```python
from build123d import *

# Parameters (mm, degrees)
SKETCH1_R               = 31.877
SKETCH1_R_2             = 2.159
BOSS_EXTRUDE1_DEPTH     = 5.08
BOSS_EXTRUDE4_START     = -5.08
BOSS_EXTRUDE4_DEPTH     = 5.08
CUT_EXTRUDE1_DEPTH      = 96.088150113
CUT_EXTRUDE1_DEPTH_BACK = 96.088150113
FILLET1_R               = 2.54


with BuildPart() as part:
    # Sketch1 → Boss-Extrude1 (new body)
    with BuildSketch(Plane.XY):
        Circle(SKETCH1_R)
        Circle(SKETCH1_R_2, mode=Mode.SUBTRACT)
        with BuildLine():
            ThreePointArc((19.487155783, 19.487155783), (-5.258505104, 27.052663549), (-25.368193256, 10.76815917))
            ThreePointArc((-25.368193256, 10.76815917), (-24.224411784, 7.937200685), (-21.393453299, 9.080982157))
            ThreePointArc((-21.393453299, 9.080982157), (-4.434591862, 22.813997371), (16.433868702, 16.433868702))
            ThreePointArc((16.433868702, 16.433868702), (19.487155783, 16.433868702), (19.487155783, 19.487155783))
        make_face(mode=Mode.SUBTRACT)
    extrude(amount=BOSS_EXTRUDE1_DEPTH)

    # Sketch2 → Boss-Extrude4 (add)
    with BuildSketch(Plane.XY.offset(5.08).offset(BOSS_EXTRUDE4_START)):
        with BuildLine():
            ThreePointArc((26.423537131, 17.830866902), (27.113483126, 16.763119094), (27.760306855, 15.668710614))
            ThreePointArc((27.760306855, 15.668710614), (28.362979586, 14.549382048), (28.920542807, 13.406913618))
            Line((28.920542807, 13.406913618), (80.920581905, 42.757221913))
            ThreePointArc((80.920581905, 42.757221913), (81.884055709, 46.217701392), (78.423576229, 47.181175196))
            Line((78.423576229, 47.181175196), (26.423537131, 17.830866902))
        make_face()
    extrude(amount=BOSS_EXTRUDE4_DEPTH)

    # Sketch6 → Cut-Extrude1 (cut, two sides: drawn at the far end of the back side and taken through both)
    # profile 1 of 2: a face of its own
    with BuildSketch(Plane.XY.offset(5.08).offset(-CUT_EXTRUDE1_DEPTH_BACK)):
        with BuildLine():
            ThreePointArc((7.239, 0), (0, -7.239), (-7.239, 0))
            Line((-7.239, 0), (-31.612710273, 4.096300546))
            ThreePointArc((-31.612710273, 4.096300546), (4.846010768, -31.506496293), (28.920542807, 13.406913618))
            Line((28.920542807, 13.406913618), (7.151828818, 1.120029266))
            ThreePointArc((7.151828818, 1.120029266), (7.217174302, 0.561708192), (7.239, 0))
        make_face()
    # profile 2 of 2: a face of its own
    with BuildSketch(Plane.XY.offset(5.08).offset(-CUT_EXTRUDE1_DEPTH_BACK)):
        with BuildLine():
            Line((-30.702053839, 8.574789739), (-5.761160237, 4.383167088))
            ThreePointArc((-5.761160237, 4.383167088), (-0.801790855, 7.194459842), (4.654823143, 5.54398255))
            Line((4.654823143, 5.54398255), (26.423537131, 17.830866902))
            ThreePointArc((26.423537131, 17.830866902), (-5.098545618, 31.466616621), (-30.702053839, 8.574789739))
        make_face()
        with BuildLine():
            ThreePointArc((-21.393453299, 9.080982157), (-24.224411784, 7.937200685), (-25.368193256, 10.76815917))
            ThreePointArc((-25.368193256, 10.76815917), (-5.258505104, 27.052663549), (19.487155783, 19.487155783))
            ThreePointArc((19.487155783, 19.487155783), (19.487155783, 16.433868702), (16.433868702, 16.433868702))
            ThreePointArc((16.433868702, 16.433868702), (-4.434591862, 22.813997371), (-21.393453299, 9.080982157))
        make_face(mode=Mode.SUBTRACT)
    extrude(amount=CUT_EXTRUDE1_DEPTH + CUT_EXTRUDE1_DEPTH_BACK, mode=Mode.SUBTRACT)

    # Fillet1
    # the kernel refuses this fillet: 2.54 mm, written as the material it adds along each edge
    with BuildSketch(Plane(origin=(7.151828818, 1.120029266, 0), x_dir=(0.8708569456123161, 0.49153655029792803, 0), z_dir=(0, 0, 1))) as fillet1_piece_1:
        with BuildLine():
            CenterArc((1.577227226, -2.54), FILLET1_R, 90, 58.70258778)
            ThreePointArc((-0.593157799, -1.220519481), (-0.267916042, -0.624189545), (0, 0))
            Line((0, 0), (1.577227226, 0))
        make_face()
    extrude(amount=5.08)
    with BuildSketch(Plane(origin=(-7.239, 0, 5.08), x_dir=(0.11271886677940961, -0.9936269204646005, 0), z_dir=(0, 0, -1))) as fillet1_piece_2:
        with BuildLine():
            CenterArc((1.918249675, 2.523812378), FILLET1_R, 196.012174579, 67.515755227)
            Line((-0.523206212, 1.823174702), (0, 0))
            ThreePointArc((0, 0), (0.815971877, 0.046134723), (1.631943753, 0))
        make_face()
    extrude(amount=5.08)
    with BuildSketch(Plane(origin=(-5.761160237, 4.383167088, 0), x_dir=(-0.9861698342812768, 0.1657379194802423, 0), z_dir=(0, 0, 1))) as fillet1_piece_3:
        with BuildLine():
            CenterArc((1.384869379, -2.54), FILLET1_R, 90, 52.834345642)
            ThreePointArc((-0.639236805, -1.005531312), (-0.298894804, -0.515940071), (0, 0))
            Line((0, 0), (1.384869379, 0))
        make_face()
    extrude(amount=5.08)
    with BuildSketch(Plane(origin=(4.654823143, 5.54398255, 0), x_dir=(-0.822747868924725, 0.5684064955468259, 0), z_dir=(0, 0, 1))) as fillet1_piece_4:
        with BuildLine():
            CenterArc((1.595093986, -2.528818084), FILLET1_R, 95.378217341, 58.70258778)
            Line((-0.689410954, -1.418576138), (0, 0))
            ThreePointArc((0, 0), (0.678510128, -0.031868462), (1.357020257, 0))
        make_face()
    extrude(amount=5.08)
    # the kernel refuses this fillet: 2.54 mm, written as the material it takes off along each edge
    with BuildSketch(Plane(origin=(-31.612710273, 4.096300546, 11.72014543), x_dir=(0.16970739547813604, 0.9854944951241623, 0), z_dir=(0, 0, -1))) as fillet1_2_piece_1:
        with BuildLine():
            CenterArc((2.550239121, 2.537794777), FILLET1_R, 179.769297531, 92.618395473)
            Line((0.010259711, 2.548022104), (0, 0))
            ThreePointArc((0, 0), (1.328029086, -0.027675553), (2.656058172, 0))
        make_face()
    extrude(amount=18.360290859, mode=Mode.SUBTRACT)
    with BuildSketch(Plane(origin=(-30.702053839, 8.574789739, 11.264732426), x_dir=(-0.23142006646754307, -0.9728539216327177, 0), z_dir=(0, 0, -1))) as fillet1_2_piece_2:
        with BuildLine():
            CenterArc((2.375331497, -2.538087003), FILLET1_R, 87.776151747, 88.383261221)
            Line((-0.158964351, -2.367956016), (0, 0))
            ThreePointArc((0, 0), (1.236946485, 0.024008109), (2.47389297, 0))
        make_face()
    extrude(amount=17.449464851, mode=Mode.SUBTRACT)


solid = part.part
```
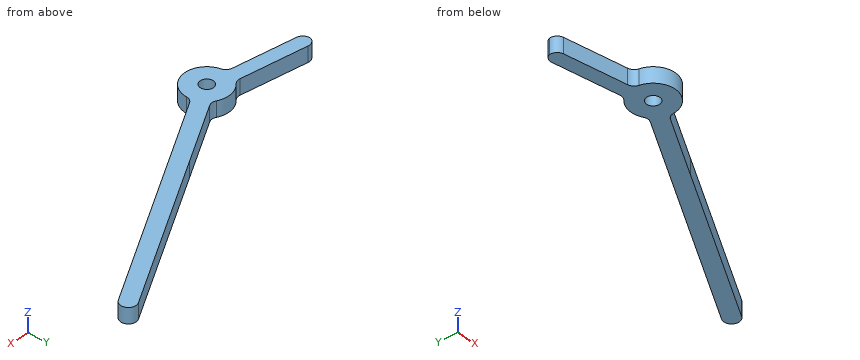
Build history of the part. All positions in model axes, mm. Coordinates: 2 decimals unless noted, no trailing zeros. Order: outer loops, then holes, each group sorted by start corner. A loop starts at its lowest first (then second) coordinate and runs counter-clockwise, first axis right, second up. Notation, with made-up numbers: (7, -13) -> (12, -13) arc R21 ccw to (12, 23) -> close; hole circle Ø2 at (89.5, -40). An arc over 180 degrees is marked (long way). Answer in a Markdown table with one row per item. Add a question column.
Q1. Band-saw the part on D-D, the plane y = 10.5. List the corners of the cut face in (x, z).
Q2. Band-saw the part on B-B, the plane z = 3.9. List the corners of the cut face in (x, y), then the cut area to 3 significant figures.
Q3. Drop flat-ended pins along their axis: pin 1 (2 mm diameter, centred on x = 58, z = 3.5, fed in from +Y); pin 2 (10 mm diameter, centred on x = -9.5, y = 12, fed in from -Z). Give the stop position or say it passes through.
Q4. Band-saw the part on C-C, the plane x = 61. List the corners of the cut face in (y, z).
Q5. Wall check: line 1 along Y through (x, z) = (0, 1.9); line 2 along X through (y, z) = (-1.5, 2); line 3 along X through (y, z) = (22.5, 1.5). Give the ranges that are in metal, low to high. Write a range as [from, to].
Q6. Band-saw the part on A-A, the plane x = 0. List the corners of the cut face in (y, z), then the cut area to 3 significant figures.
Answers follow:
| question | item | result |
|---|---|---|
| 1 | outline | (13.44, 0) -> (23.77, 0) -> (23.77, 5.08) -> (13.44, 5.08) -> close |
| 2 | outline | (-31.21, 6.44) arc R2.54 ccw to (-29.1, 3.67) -> (-9.11, 0.31) arc R2.54 cw to (-7.06, -1.62) arc R7.24 ccw to (7.24, -0.23) arc R2.54 cw to (8.53, 1.9) -> (80.92, 42.76) arc R2.54 ccw to (78.42, 47.18) -> (6.03, 6.32) arc R2.54 cw to (3.54, 6.32) arc R7.24 ccw to (-4.96, 5.27) arc R2.54 cw to (-7.13, 4.61) -> (-28.36, 8.18) arc R2.54 ccw to start; hole circle Ø4.32 at (0, 0) |
| 2 | area | 701 mm^2 |
| 3 | pin 1 | y = 36.22 |
| 3 | pin 2 | through |
| 4 | outline | (31.51, 0) -> (37.35, 0) -> (37.35, 5.08) -> (31.51, 5.08) -> close |
| 5 | line 1 | [-7.24, -2.16], [2.16, 7.24] |
| 5 | line 2 | [-7.09, -1.55], [1.55, 7.08] |
| 5 | line 3 | [34.7, 45.03] |
| 6 | outline | (-7.24, 0) -> (-2.16, 0) -> (-2.16, 5.08) -> (-7.24, 5.08) -> close; (2.16, 0) -> (7.24, 0) -> (7.24, 5.08) -> (2.16, 5.08) -> close |
| 6 | area | 51.6 mm^2 |
